Geometry: final body of the model. Coordinates: model frame, mm. Round coordinates to 2 decimals unless told otherwise and drop trailing zeros. Write each loop counter-clockwise with the first axis right and the second up, starting at its lowest first coordinate (ties: lowest second). Pieces come first, ordered by that corner, then holes. Notation, with made-up numbers: M 6,76.25 L 18,76.25 A20 ccw 18,105.25 Z; hole C 77.5,54 d11. An arc over 180 degrees is marked long. Use one line per item in the form item = value. Start each with the question number.
Item 1: Pin query (flat end, axial travel): pin 1 Ø12 at (y, z) = (-6.5, 17.5) entering from +X; pin 2 Ø5 at (x, y) = (-6, -6.5) entering from +Z; pin 3 Ø10 at (y, z) = (7.5, 17.5) entering from -X. Return the tip coordinate at first contact, or that it passes through.
Item 2: Section query A-A (z = 15.25). Return loops of the section in (x, y), and give its area (3 significant figures).
Item 3: Pull-direction query (X, two-part tool) for faces 1 (the cylindrical face through (-1.08, -4.88, 10.89)), 2 (the flat face through (3, -6, 2)), 3 (the cylindrical face through (0, -2, 11)); classes: pulls with the +X half, pulls with the -X half, needs draft (parallel to the pull), parting line crosses it, or undercut.
Item 4: Ray query, probe 1 along Y at (x, z) = (0, 7); probe 2 along Z at (x, y) = (-5.5, -5); probe 3 along Y at (x, z) = (-1, 17). Return the intervals inside material, ascending.
from build123d import *

# Parameters (mm, degrees)
SKETCH1_R           = 15
BOSS_EXTRUDE1_DEPTH = 2
SKETCH2_R           = 5
BOSS_EXTRUDE2_DEPTH = 18
SKETCH3_RX          = 2.7
SKETCH3_RY          = 2.2
CUT_EXTRUDE1_DEPTH  = 3
SKETCH4_R           = 2
CUT_EXTRUDE2_DEPTH  = 30
FILLET2_R           = 1
CHAMFER1_SIZE       = 1
FILLET3_R           = 1
FILLET4_R           = 1
FILLET6_R           = 1


with BuildPart() as part:
    # Sketch1 → Boss-Extrude1 (new body)
    with BuildSketch(Plane.XY):
        Circle(SKETCH1_R)
    extrude(amount=BOSS_EXTRUDE1_DEPTH)

    # Sketch2 → Boss-Extrude2 (add)
    with BuildSketch(Plane.XY.offset(2)):
        Circle(SKETCH2_R)
    extrude(amount=BOSS_EXTRUDE2_DEPTH)

    # Sketch3 → Cut-Extrude1 (cut)
    with BuildSketch(Plane(origin=(0, 0, 0), x_dir=(-1, 0, 0), z_dir=(0, 0, -1))):
        with Locations(Location((0, 0), (0, 0, 0))):
            Ellipse(SKETCH3_RX, SKETCH3_RY)
    extrude(amount=-CUT_EXTRUDE1_DEPTH, mode=Mode.SUBTRACT)

    # Sketch4 → Cut-Extrude2 (cut)
    with BuildSketch(Plane(origin=(0, 0, 0), x_dir=(-1, 0, 0), z_dir=(0, 0, -1))):
        Circle(SKETCH4_R)
    extrude(amount=-CUT_EXTRUDE2_DEPTH, mode=Mode.SUBTRACT)

    # Fillet2
    fillet2_edges = [part.edges().sort_by_distance(p)[0] for p in [
        (2.699999981, -0.000263168, 0),
    ]]
    fillet(fillet2_edges, radius=FILLET2_R)

    # Chamfer1
    chamfer1_edges = [part.edges().sort_by_distance(p)[0] for p in [
        (-5, 0, 2),
    ]]
    chamfer(chamfer1_edges, length=CHAMFER1_SIZE)

    # Fillet3
    fillet3_edges = [part.edges().sort_by_distance(p)[0] for p in [
        (-15, 0, 2),
    ]]
    fillet(fillet3_edges, radius=FILLET3_R)

    # Fillet4
    fillet4_edges = [part.edges().sort_by_distance(p)[0] for p in [
        (-5, 0, 20),
    ]]
    fillet(fillet4_edges, radius=FILLET4_R)

    # Fillet6
    fillet6_edges = [part.edges().sort_by_distance(p)[0] for p in [
        (2, 0, 20),
    ]]
    fillet(fillet6_edges, radius=FILLET6_R)


solid = part.part
Working result:
q1.pin_1 = 4.97
q1.pin_2 = 2
q1.pin_3 = -4.33
q2.outline = C 0,0 d10; hole C 0,0 d4
q2.area = 66.0 mm²
q3.face_1 = parting line crosses it
q3.face_2 = needs draft
q3.face_3 = undercut
q4.probe_1 = -5 to -2, 2 to 5
q4.probe_2 = 0 to 2
q4.probe_3 = -4.9 to -1.73, 1.73 to 4.9
